Verification items for the finished model (mm, model axes). Round coordinates to 2 decimals unless told otherwise and drop trailing zeros. Write each loop counter-clockwise with the first axis right and the second up, starting at its lowest first coordinate (ties: lowest second). Pieces come first, ordered by that corner, then holes. Notation, with made-up numbers: (-9.5, 83) - (2.5, 83) arc R18 cw to (2.5, 102) - close; hole circle Ø11 at (28.5, 87). An arc over 180 degrees is marked (long way). Answer as a JSON object with one key per item and string values.
```python
from build123d import *

# Parameters (mm, degrees)
BASE_FLANGE1_DEPTH = 817
SKETCH6_R          = 10
CUT_EXTRUDE1_DEPTH = 10


# Sheet-metal steps are written as plain solids
with BuildPart() as part:
    # Sketch1 → Base-Flange1 (new body)
    with BuildSketch(Plane.XY):
        with BuildLine():
            Line((12, 0), (4, 0))
            ThreePointArc((4, 0), (1.171572875, 1.171572875), (0, 4))
            Line((0, 4), (0, 10))
            ThreePointArc((0, 10), (1.171572875, 12.828427125), (4, 14))
            Line((4, 14), (161, 14))
            ThreePointArc((161, 14), (163.828427125, 12.828427125), (165, 10))
            Line((165, 10), (165, 4))
            ThreePointArc((165, 4), (163.828427125, 1.171572875), (161, 0))
            Line((161, 0), (153, 0))
            Line((153, 0), (153, 0.8))
            Line((153, 0.8), (161, 0.8))
            ThreePointArc((161, 0.8), (163.2627417, 1.7372583), (164.2, 4))
            Line((164.2, 4), (164.2, 10))
            ThreePointArc((164.2, 10), (163.2627417, 12.2627417), (161, 13.2))
            Line((161, 13.2), (4, 13.2))
            ThreePointArc((4, 13.2), (1.7372583, 12.2627417), (0.8, 10))
            Line((0.8, 10), (0.8, 4))
            ThreePointArc((0.8, 4), (1.7372583, 1.7372583), (4, 0.8))
            Line((4, 0.8), (12, 0.8))
            Line((12, 0.8), (12, 0))
        make_face()
    extrude(amount=BASE_FLANGE1_DEPTH)

    # Sketch6 → Cut-Extrude1 (cut)
    with BuildSketch(Plane(origin=(0, 14, 0), x_dir=(1, 0, 0), z_dir=(0, 1, 0))):
        with Locations(Location((107.5, -326, 0), (0, 0, 270))):
            Circle(SKETCH6_R)
        with Locations(Location((107.5, -161, 0), (0, 0, 270))):
            Circle(SKETCH6_R)
        with Locations(Location((107.5, -491, 0), (0, 0, 270))):
            Circle(SKETCH6_R)
        with Locations(Location((107.5, -656, 0), (0, 0, 270))):
            Circle(SKETCH6_R)
        with Locations(Location((57.5, -656, 0), (0, 0, 270))):
            Circle(SKETCH6_R)
        with Locations(Location((57.5, -491, 0), (0, 0, 270))):
            Circle(SKETCH6_R)
        with Locations(Location((57.5, -326, 0), (0, 0, 270))):
            Circle(SKETCH6_R)
        with Locations(Location((57.5, -161, 0), (0, 0, 270))):
            Circle(SKETCH6_R)
    extrude(amount=-CUT_EXTRUDE1_DEPTH, mode=Mode.SUBTRACT)


solid = part.part
```
1. Cross-section at A-A (x = 107.5). Record the boundary of the cut face in (y, z), plus the area to 3 significant figures.
Completed:
{"outline": "(13.2, 0) - (14, 0) - (14, 151) - (13.2, 151) - close; (13.2, 171) - (14, 171) - (14, 316) - (13.2, 316) - close; (13.2, 336) - (14, 336) - (14, 481) - (13.2, 481) - close; (13.2, 501) - (14, 501) - (14, 646) - (13.2, 646) - close; (13.2, 666) - (14, 666) - (14, 817) - (13.2, 817) - close", "area": "590 mm^2"}
2. Cross-section at C-C (z = 550). Record the boundary of the cut face in (x, y), plus the area to 3 significant figures.
Completed:
{"outline": "(0, 4) arc R4 ccw to (4, 0) - (12, 0) - (12, 0.8) - (4, 0.8) arc R3.2 cw to (0.8, 4) - (0.8, 10) arc R3.2 cw to (4, 13.2) - (161, 13.2) arc R3.2 cw to (164.2, 10) - (164.2, 4) arc R3.2 cw to (161, 0.8) - (153, 0.8) - (153, 0) - (161, 0) arc R4 ccw to (165, 4) - (165, 10) arc R4 ccw to (161, 14) - (4, 14) arc R4 ccw to (0, 10) - close", "area": "166 mm^2"}
3. Go/stop test with flat-tipped pins: pin 1 (1.5 mm diameter, centred on x = 85.5, y = 11, fed in from +Z); pin 2 (23 mm diameter, centred on x = 57.5, z = 491, fed in from -Y); pin 3 (3 mm diameter, centred on y = 2, z = 262, fed in from -X); pin 4 (23 mm diameter, centred on x = 107.5, z = 491, fed in from +Y). Record where each tip stops, or that it passes through.
Completed:
{"pin 1": "passes through", "pin 2": "stops at y = 13.2", "pin 3": "stops at x = 0.03", "pin 4": "stops at y = 14"}
4. Material ranges on probe 1 along Y at (x, z) = (154.5, 783); probe 2 along X at (y, z) = (13.55, 656); probe 3 along X at (y, z) = (13.5, 656), recorded low to high. Write a range as from..to.
Completed:
{"probe 1": "y = 0..0.8, 13.2..14", "probe 2": "x = 2.16..47.5, 67.5..97.5, 117.5..162.84", "probe 3": "x = 2.06..47.5, 67.5..97.5, 117.5..162.94"}
5. Cross-section at B-B (z = 161). Record the boundary of the cut face in (x, y).
Completed:
{"outline": "(0, 4) arc R4 ccw to (4, 0) - (12, 0) - (12, 0.8) - (4, 0.8) arc R3.2 cw to (0.8, 4) - (0.8, 10) arc R3.2 cw to (4, 13.2) - (47.5, 13.2) - (47.5, 14) - (4, 14) arc R4 ccw to (0, 10) - close; (67.5, 13.2) - (97.5, 13.2) - (97.5, 14) - (67.5, 14) - close; (117.5, 13.2) - (161, 13.2) arc R3.2 cw to (164.2, 10) - (164.2, 4) arc R3.2 cw to (161, 0.8) - (153, 0.8) - (153, 0) - (161, 0) arc R4 ccw to (165, 4) - (165, 10) arc R4 ccw to (161, 14) - (117.5, 14) - close"}
6. Mould release check, pull along X, two halves, no side actions. Record for faces 1 (the face through (107.94, 13.61, 316.01)), 2 (the face through (60.5, 13.61, 500.54)), 3 (the face through (81, 14, 403)): released by +X, released by -X, zero draft, split by the parting line, or undercut.
Completed:
{"face 1": "undercut", "face 2": "undercut", "face 3": "zero draft"}
